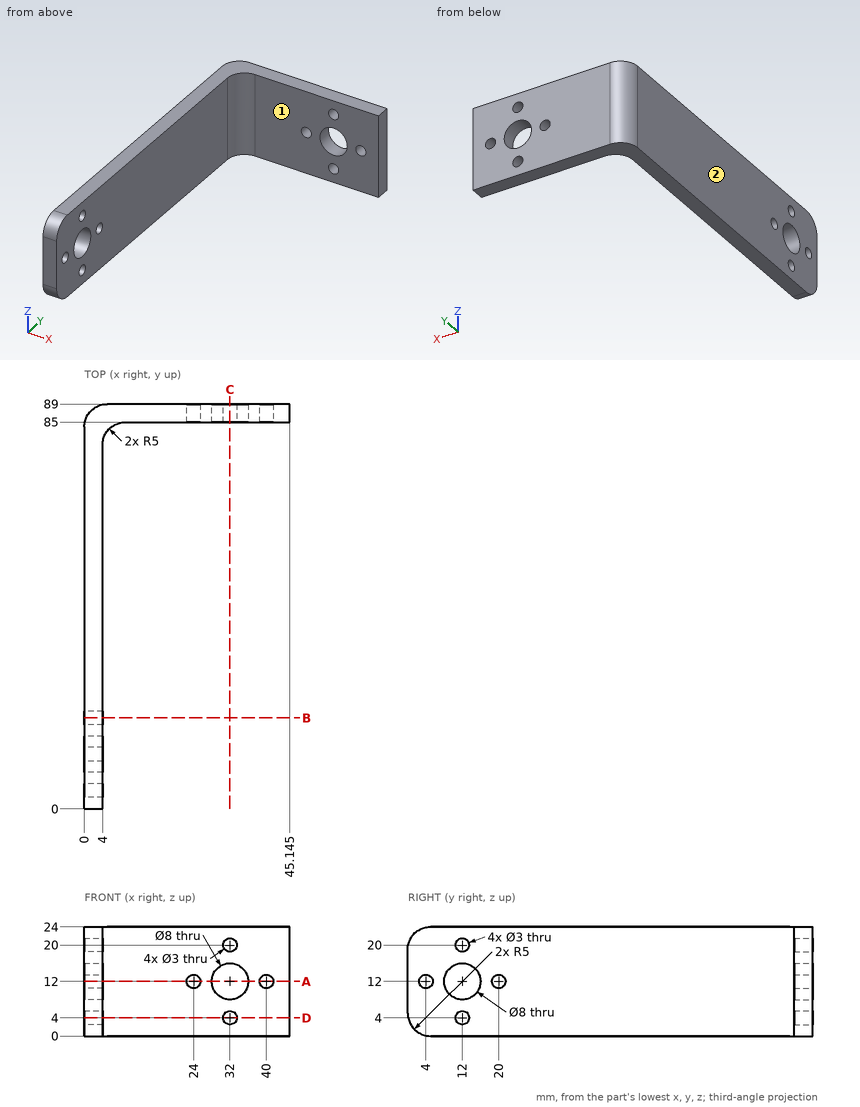
Print and shaded views of the part. All mm, measured from the part's lowest x, y and z. A direction names the side the tool comes from. Round coordinates to 2 decimals unless told otherwise and drop trailing zeros. Write each loop counter-clockwise with the first axis right and the second up, starting at its lowest first coordinate (ties: lowest second). Pieces come first, ordered by that corner, then holes. Notation, with made-up numbers: (-2.75, 7.5) -> (37.25, 7.5) arc R29 cw to (37.25, 39.5) -> close; hole circle Ø4 at (76, 53.5). An arc over 180 degrees is marked (long way). Answer in a Markdown table with one row per item. Add a question column.
Item 1: Saw through at D-D, the plane z = 4. Write the cut outline in (x, y) (1 decimal), then the cut area to 3 significant figures.
Item 2: Saw through at A-A, the plane z = 12. Count the separate pieces of the cut face and the enclosed holes in it.
Item 3: Saw through at C-C, the plane x = 32. Write the cut outline in (y, z), then the cut area to 3 significant figures.
Item 4: Drill centre lines: line 1 (Z direction, x = 40, y = 87); line 2 (Y direction, x = 3.05, z = 12); line 3 (X direction, y = 87.4, z = 12) (1 decimal). Where is each one in solid material? Low to high. Write a range as from..to.
Item 5: Which spindle directions (+Z, -Z, +X, -X, +Y, -Y) get a long thin tool onto all of the face, cutting with end or side? Do the marked faces 1 and 2. Say none if no direction does.
Item 6: Saw through at B-B, the plane y = 20. Write the cut outline in (x, z).
Item 7: Drop flat-ended pins along their axis: pin 1 Ø8 at (x, z) = (22.5, 9.5) entering from -Y; pin 2 Ø7 at (y, z) = (27, 6.5) entering from +X. Give the stop position or say it passes through.
Findings below:
| question | item | result |
|---|---|---|
| 1 | outline | (0, 0.1) -> (4, 0.1) -> (4, 10.5) -> (0, 10.5) -> close; (0, 13.5) -> (4, 13.5) -> (4, 80) arc R5 cw to (9, 85) -> (30.5, 85) -> (30.5, 89) -> (5, 89) arc R5 ccw to (0, 84) -> close; (33.5, 85) -> (45.1, 85) -> (45.1, 89) -> (33.5, 89) -> close |
| 1 | area | 496 mm^2 |
| 2 | separate pieces | 7 |
| 2 | enclosed holes | 0 |
| 3 | outline | (85, 0) -> (89, 0) -> (89, 2.5) -> (85, 2.5) -> close; (85, 5.5) -> (89, 5.5) -> (89, 8) -> (85, 8) -> close; (85, 16) -> (89, 16) -> (89, 18.5) -> (85, 18.5) -> close; (85, 21.5) -> (89, 21.5) -> (89, 24) -> (85, 24) -> close |
| 3 | area | 40.0 mm^2 |
| 4 | line 1 | z = 0..10.5, 13.5..24 |
| 4 | line 2 | y = 0..2.5, 5.5..8, 16..18.5, 21.5..88.6 |
| 4 | line 3 | x = 1.3..22.5, 25.5..28, 36..38.5, 41.5..45.1 |
| 5 | face 1 | +Z, -Z, +X, -Y |
| 5 | face 2 | +Z, -Z, -X, +Y, -Y |
| 6 | outline | (0, 0) -> (4, 0) -> (4, 10.5) -> (0, 10.5) -> close; (0, 13.5) -> (4, 13.5) -> (4, 24) -> (0, 24) -> close |
| 7 | pin 1 | stops at y = 85 |
| 7 | pin 2 | stops at x = 4 |
